Read the model definition and answer for the solid it produces. Units are mm, in the model's axes. A direction names the side the tool comes from. Coordinates: 2 decimals unless noted, no trailing zeros. Write each loop counter-clockwise with the first axis right and the second up, starting at its lowest first coordinate (ties: lowest second). Pieces come first, ordered by that corner, then holes. Notation, with made-up numbers: (83.5, -24.5) - (134.5, -24.5) arc R19 ccw to (134.5, -3.5) - close; hole circle Ø2 at (-29.5, 51.5). An arc over 180 degrees is marked (long way). Use a Markdown table: item, result.
from build123d import *

# Parameters (mm, degrees)
SKETCH1_W           = 49
SKETCH1_H           = 54
BOSS_EXTRUDE1_DEPTH = 2.5
SKETCH2_W           = 55
SKETCH2_H           = 60
BOSS_EXTRUDE2_DEPTH = 5
FILLET1_R           = 5


with BuildPart() as part:
    # Sketch1 → Boss-Extrude1 (new body)
    with BuildSketch(Plane(origin=(0, 0, 0), x_dir=(1, 0, 0), z_dir=(0, 1, 0))):
        Rectangle(SKETCH1_W, SKETCH1_H)
    extrude(amount=BOSS_EXTRUDE1_DEPTH)

    # Sketch2 → Boss-Extrude2 (add)
    with BuildSketch(Plane.XZ):
        Rectangle(SKETCH2_W, SKETCH2_H)
    extrude(amount=BOSS_EXTRUDE2_DEPTH)

    # Fillet1
    fillet1_edges = [part.edges().sort_by_distance(p)[0] for p in [
        (-27.5, -2.5, 30),
        (-27.5, -2.5, -30),
        (27.5, -2.5, -30),
        (27.5, -2.5, 30),
        (-27.5, -5, 0),
        (0, -5, -30),
        (27.5, -5, 0),
        (0, -5, 30),
    ]]
    fillet(fillet1_edges, radius=FILLET1_R - 0.0001)  # a hair under: the kernel refuses the full size


solid = part.part
(1) For faces 1 (the flat face through (24.5, 1, 0)), 2 (the flat face through (0, 1, -27)), 3 (the flat face through (0, 1, 27)), determine the directions among +Z, -Z, +X, -X, +Y, -Y from which every point of the face is accessible in a straight line to the end or side of a thin tool.
Report:
| item | result |
|---|---|
| face 1 | +Z, -Z, +X, +Y |
| face 2 | -Z, +X, -X, +Y |
| face 3 | +Z, +X, -X, +Y |
(2) Each of these flat-tipped pins is pushed along its axis until it touches: P1, Ø1.5, axis at y = -3, z = -8.5, coming from the +X side; P2, Ø0.8, axis at x = 2.5, y = 1.5, coming from the +Z side; P3, Ø2, axis at y = -4, z = 9.5, coming from the +X side. Where does it stop, or does it pass through?
Report:
| item | result |
|---|---|
| P1 | stops at x = 26.97 |
| P2 | stops at z = 27 |
| P3 | stops at x = 26.5 |
(3) A cutting plane is placed at C-C, the plane y = -4. Write down the section's boundary in (x, z).
Report:
| item | result |
|---|---|
| outline | (-25.5, -25) arc R3 ccw to (-22.5, -28) - (22.5, -28) arc R3 ccw to (25.5, -25) - (25.5, 25) arc R3 ccw to (22.5, 28) - (-22.5, 28) arc R3 ccw to (-25.5, 25) - close |
(4) Straight lines are drawn through the part: L1, parallel to X at y = 1.5, z = 9.5; L2, parallel to Z at x = 15.5, y = 2; L3, parallel to Z at x = -4.5, y = -2. For each, find the intervals that lie inside material, in ascending order.
Report:
| item | result |
|---|---|
| L1 | x = -24.5 to 24.5 |
| L2 | z = -27 to 27 |
| L3 | z = -29.58 to 29.58 |
(5) A cutting plane is placed at D-D, the plane y = 1.75. Write down the section's boundary in (x, z), and give its area (3 significant figures).
Report:
| item | result |
|---|---|
| outline | (-24.5, -27) - (24.5, -27) - (24.5, 27) - (-24.5, 27) - close |
| area | 2,650 mm² |
